For this review, take the finished solid that the model builds, in its own axes (mm). Face numbers are marked on the shaded views. A direction names the side the tool comes from. Give positions to 0.01 mm unless a question says otherwise; leave off trailing zeros. Write each loop counter-clockwise with the first axis right and the second up, starting at its lowest first coordinate (ties: lowest second). Pieces come first, ordered by that corner, then holes. Notation, with made-up numbers: (19.25, 82.5) -> (53.25, 82.5) arc R12 cw to (53.25, 94.5) -> close; hole circle Ø6 at (-5, 29.25). An arc over 180 degrees is marked (long way). Return JSON: item names as keys, results as strings.
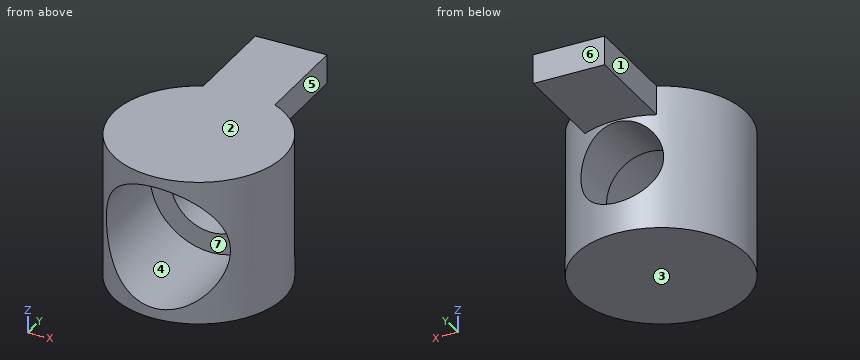
from build123d import *

# Parameters (mm, degrees)
SKETCH_1_W          = 7.8
SKETCH_1_H          = 28.46
EXTRUDE_1_DEPTH     = 3.2
SKETCH_4_W          = 7.8
SKETCH_4_H          = 7.178435562
CUT_EXTRUDE_1_DEPTH = 16.097777982
SKETCH_2_R          = 9.25
EXTRUDE_2_DEPTH     = 15.8
SKETCH_5_R          = 4.5
CUT_EXTRUDE_2_DEPTH = 33.469895288
SKETCH_6_R          = 6.75
CUT_EXTRUDE_3_DEPTH = 12


with BuildPart() as part:
    # 草图1 → 凸台-拉伸1 (new body)
    with BuildSketch(Plane.XY):
        Rectangle(SKETCH_1_W, SKETCH_1_H)
    extrude(amount=EXTRUDE_1_DEPTH)

    # 草图4 → 切除-拉伸1 (cut, through all)
    with BuildSketch(Plane(origin=(0, 0, 0), x_dir=(-1, 0, 0), z_dir=(0, 0, -1))):
        with Locations((0, -10.640782219)):
            Rectangle(SKETCH_4_W, SKETCH_4_H)
    extrude(amount=-CUT_EXTRUDE_1_DEPTH, mode=Mode.SUBTRACT)

    # 草图2 → 凸台-拉伸2 (add)
    with BuildSketch(Plane.XY.offset(3.2)):
        with Locations((0, -4.98)):
            Circle(SKETCH_2_R)
    extrude(amount=-EXTRUDE_2_DEPTH)

    # 草图5 → 切除-拉伸2 (cut, through all)
    with BuildSketch(Plane(origin=(0, 14.23, 0), x_dir=(1, 0, 0), z_dir=(0, 1, 0))):
        with Locations(Location((0, 4.7, 0), (0, 0, 270))):
            Circle(SKETCH_5_R)
    extrude(amount=-CUT_EXTRUDE_2_DEPTH, mode=Mode.SUBTRACT)

    # 草图6 → 切除-拉伸3 (cut)
    with BuildSketch(Plane(origin=(0, -14.23, 0), x_dir=(-1, 0, 0), z_dir=(0, 1, 0))):
        with Locations(Location((0, -4.7, 0), (0, 0, 270))):
            Circle(SKETCH_6_R)
    extrude(amount=CUT_EXTRUDE_3_DEPTH, mode=Mode.SUBTRACT)


solid = part.part
1. The part is to be moulded in two halves that separate along Z. For the marked faces 1, 2, 3 and 4, say which applies: +Z half, -Z half, draft (parallel to the pull), parting line (faces both ways), or undercut.
Results found:
{"face 1": "draft", "face 2": "+Z half", "face 3": "-Z half", "face 4": "undercut"}
2. Add section A-A, the plane x = 0. State the section outline as (y, z) points, plus the area to 3 significant figures.
Results found:
{"outline": "(-14.23, -12.6) -> (4.27, -12.6) -> (4.27, -9.2) -> (-2.23, -9.2) -> (-2.23, -11.45) -> (-14.23, -11.45) -> close; (-14.23, 2.05) -> (-2.23, 2.05) -> (-2.23, -0.2) -> (4.27, -0.2) -> (4.27, 0) -> (14.23, 0) -> (14.23, 3.2) -> (-14.23, 3.2) -> close", "area": "104 mm²"}
3. For the marked faces 5, 6 and 7, list the 3-axis set-ups (+Z, -Z, +X, -X, +Y, -Y) from which the entire face can be reached by the end or side of a thin tool; tool diameter is ignored.
Results found:
{"face 5": "+Z, -Z, +X, +Y", "face 6": "+Z, -Z, +X, -X, +Y", "face 7": "-Y"}
4. For pin 1 (8 mm diameter, centred on x = -6, z = -10, fed in from -Y); pin 2 (2.5 mm diameter, centred on x = 1.5, y = 7, fed in from -Z); pin 3 (5 mm diameter, centred on y = 5, z = -8, fed in from -X), all flat-tipped, find the tip position at first contact; note any pin that passes through.
Results found:
{"pin 1": "stops at y = -13.98", "pin 2": "stops at z = 0", "pin 3": "stops at x = -5.44"}
5. To check wall thickness, follow probe 1 along Z at (x, y) = (0, 1); probe 2 along X at (y, z) = (2, -4.7); probe 3 along X at (y, z) = (1.25, -3.5). State the ranges of each line that lie inside material, in increasing order.
Results found:
{"probe 1": "z = -12.6 to -9.2, -0.2 to 3.2", "probe 2": "x = -6.07 to -4.5, 4.5 to 6.07", "probe 3": "x = -6.84 to -4.34, 4.34 to 6.84"}
6. Add section C-C, the plane y = -4.98. State the section outline as (x, z) points, plus the area to 3 significant figures.
Results found:
{"outline": "(-9.25, -12.6) -> (9.25, -12.6) -> (9.25, 3.2) -> (-9.25, 3.2) -> close; hole circle Ø13.5 at (0, -4.7)", "area": "149 mm²"}
7. Add section B-B, the plane z = -1.5. State the section outline as (x, y) points.
Results found:
{"outline": "(-5.94, -12.07) -> (-5.94, -2.23) -> (-3.16, -2.23) -> (-3.16, 3.71) arc R9.25 ccw to start; (3.16, -2.23) -> (5.94, -2.23) -> (5.94, -12.07) arc R9.25 ccw to (3.16, 3.71) -> close"}
8. Add section D-D, the plane x = 2.5. State the section outline as (y, z) points.
Results found:
{"outline": "(-13.89, -12.6) -> (3.93, -12.6) -> (3.93, -8.44) -> (-2.23, -8.44) -> (-2.23, -10.97) -> (-13.89, -10.97) -> close; (-13.89, 1.57) -> (-2.23, 1.57) -> (-2.23, -0.96) -> (3.93, -0.96) -> (3.93, 0) -> (14.23, 0) -> (14.23, 3.2) -> (-13.89, 3.2) -> close"}
